CAD build for the part. Positions are in the model's coordinates, mm. A direction names the side the tool comes from. Round coordinates to 2 decimals unless told otherwise and drop trailing zeros. Write each loop counter-clockwise with the first axis right and the second up, starting at its lowest first coordinate (ties: lowest second). Pieces come first, ordered by that corner, then holes. Notation, with made-up numbers: M 70.5,32 L 80.5,32 A23 ccw 80.5,62 Z; hole C -14,71.5 d7. An arc over 180 degrees is marked long. Write each question's results on one line, items separated by ' | '. Start each with the question number.
```python
from build123d import *

# Parameters (mm, degrees)
SKETCH1_W           = 200
SKETCH1_H           = 120
BOSS_EXTRUDE1_DEPTH = 5
SKETCH2_W           = 12.5
SKETCH2_H           = 56.72
BOSS_EXTRUDE2_DEPTH = 28.82
SKETCH3_W           = 20.22
SKETCH3_H           = 40.72
CUT_EXTRUDE1_DEPTH  = 28.82
SKETCH4_W           = 8.8
SKETCH4_H           = 8.8
CUT_EXTRUDE2_DEPTH  = 19.82
MIRROR1_START       = 5
MIRROR1_OUTLINE_W   = 25
MIRROR1_OUTLINE_H   = 56.72
MIRROR1_OUTLINE_W_2 = 20.22
MIRROR1_OUTLINE_H_2 = 40.72
MIRROR1_DEPTH       = 28.82
SKETCH5_W           = 8.8
SKETCH5_H           = 8.8
CUT_EXTRUDE3_DEPTH  = 19.82


# Read off the part's stored shape, not the designer's step: Mirror1
with BuildPart() as part:
    # Sketch1 → Boss-Extrude1 (new body)
    with BuildSketch(Plane.XY):
        Rectangle(SKETCH1_W, SKETCH1_H)
    extrude(amount=BOSS_EXTRUDE1_DEPTH)

    # Sketch2 → Boss-Extrude2 (add)
    with BuildSketch(Plane.XY.offset(5)):
        with Locations((-6.25, 31.64)):
            Rectangle(SKETCH2_W, SKETCH2_H)
        with Locations((6.25, 31.64)):
            Rectangle(SKETCH2_W, SKETCH2_H)
    extrude(amount=BOSS_EXTRUDE2_DEPTH)

    # Sketch3 → Cut-Extrude1 (cut)
    with BuildSketch(Plane.XY.offset(33.82)):
        with Locations((0, 31.64)):
            Rectangle(SKETCH3_W, SKETCH3_H)
    extrude(amount=-CUT_EXTRUDE1_DEPTH, mode=Mode.SUBTRACT)

    # Sketch4 → Cut-Extrude2 (cut)
    with BuildSketch(Plane.XZ.offset(-52)):
        with Locations((0, 9.4)):
            Rectangle(SKETCH4_W, SKETCH4_H)
    extrude(amount=-CUT_EXTRUDE2_DEPTH, mode=Mode.SUBTRACT)

    # Mirror1 outline → Mirror1 (add)
    with BuildSketch(Plane.XY.offset(MIRROR1_START)):
        with Locations((0, -31.64)):
            Rectangle(MIRROR1_OUTLINE_W, MIRROR1_OUTLINE_H)
        with Locations((0, -31.64)):
            Rectangle(MIRROR1_OUTLINE_W_2, MIRROR1_OUTLINE_H_2, mode=Mode.SUBTRACT)
    extrude(amount=MIRROR1_DEPTH)

    # Sketch5 → Cut-Extrude3 (cut)
    with BuildSketch(Plane(origin=(0, -52, 0), x_dir=(1, 0, 0), z_dir=(0, 1, 0))):
        with Locations((0, -9.4)):
            Rectangle(SKETCH5_W, SKETCH5_H)
    extrude(amount=-CUT_EXTRUDE3_DEPTH, mode=Mode.SUBTRACT)


solid = part.part
```
1) Saw through at B-B, the plane z = 7.5. Write the cut outline in (x, y).
2) Pull direction Y, two halves, no side cores. Call faces 1 (the face through (0, 11.28, 20)), 2 (the face through (0, -60, 4)), 3 (the face through (-1, 1, 0)): pulls with the +Y half, pulls with the -Y half, needs draft (parallel to the pull), parting line crosses it, or undercut.
3) Drop flat-ended pins along their axis: pin 1 Ø14.5 at (y, z) = (-35, 21) entering from -X; pin 2 Ø6 at (x, y) = (5, 24) entering from +Z. Give the stop position or say it passes through.
4) Saw through at A-A, the plane z = 18.5. Write the cut outline in (x, y).
5) Saw through at D-D, the plane x = 74.5. Write the cut outline in (y, z).
6) Wall check: line 1 along X through (y, z) = (44.5, 17.5); line 2 along Z through (x, y) = (78.5, -16); line 3 along X through (y, z) = (-6.5, 14). Give the ranges that are in metal, low to high. Write a range as from..to.
7) 3-axis set-ups, long thin cutter, end or side, ignore diameter. For faces 4 (the face through (0, 60, 4)), 5 (the face through (0, 3.28, 19)), 6 (the face through (0, 56, 13.8)), 7 (the face through (4.4, -56, 9)), 8 (the face through (0, -52, 22)): which of +Z, -Z, +X, -X, +Y, -Y reach the whole face in a straight line?
8) Saw through at C-C, the plane y = 35. Write the cut outline in (x, z), plus the area to 3 significant figures.
Filled sheet:
1) outline: M -12.5,-60 L -4.4,-60 L -4.4,-52 L -10.11,-52 L -10.11,-11.28 L 10.11,-11.28 L 10.11,-52 L 4.4,-52 L 4.4,-60 L 12.5,-60 L 12.5,-3.28 L -12.5,-3.28 Z; M -12.5,3.28 L 12.5,3.28 L 12.5,60 L 4.4,60 L 4.4,52 L 10.11,52 L 10.11,11.28 L -10.11,11.28 L -10.11,52 L -4.4,52 L -4.4,60 L -12.5,60 Z
2) face 1: undercut | face 2: pulls with the -Y half | face 3: needs draft
3) pin 1: stops at x = -12.5 | pin 2: stops at z = 5
4) outline: M -12.5,-60 L 12.5,-60 L 12.5,-3.28 L -12.5,-3.28 Z; M -12.5,3.28 L 12.5,3.28 L 12.5,60 L -12.5,60 Z; hole M -10.11,-52 L 10.11,-52 L 10.11,-11.28 L -10.11,-11.28 Z; hole M -10.11,11.28 L 10.11,11.28 L 10.11,52 L -10.11,52 Z
5) outline: M -60,0 L 60,0 L 60,5 L -60,5 Z
6) line 1: x = -12.5..-10.11, 10.11..12.5 | line 2: z = 0..5 | line 3: x = -12.5..12.5
7) face 4: +Z, -Z, +X, -X, +Y | face 5: +Z, +X, -X | face 6: +Y | face 7: -Y | face 8: +Z
8) outline: M -100,0 L 100,0 L 100,5 L 12.5,5 L 12.5,33.82 L 10.11,33.82 L 10.11,5 L -10.11,5 L -10.11,33.82 L -12.5,33.82 L -12.5,5 L -100,5 Z | area: 1,140 mm^2
